```python
from build123d import *

# Parameters (mm, degrees)
SKETCH1_R           = 2.75
BOSS_EXTRUDE1_DEPTH = 6.35
FILLET1_R           = 6.35
CHAMFER1_SIZE       = 3.175


with BuildPart() as part:
    # Sketch1 → Boss-Extrude1 (new body)
    with BuildSketch(Plane.XY):
        with BuildLine():
            ThreePointArc((-19.05, 19.05), (-31.75, 6.35), (-19.05, -6.35))
            Line((-19.05, -6.35), (-19.05, -260.35))
            ThreePointArc((-19.05, -260.35), (-31.75, -273.05), (-19.05, -285.75))
            Line((-19.05, -285.75), (241.3, -285.75))
            ThreePointArc((241.3, -285.75), (254, -273.05), (241.3, -260.35))
            Line((241.3, -260.35), (241.3, -6.35))
            ThreePointArc((241.3, -6.35), (254, 6.35), (241.3, 19.05))
            Line((241.3, 19.05), (-19.05, 19.05))
        make_face()
        with Locations((241.3, 6.35)):
            Circle(SKETCH1_R, mode=Mode.SUBTRACT)
        with Locations((-19.05, -273.05)):
            Circle(SKETCH1_R, mode=Mode.SUBTRACT)
        with Locations((-9.525, -276.225)):
            Circle(SKETCH1_R, mode=Mode.SUBTRACT)
        with Locations((231.775, -276.225)):
            Circle(SKETCH1_R, mode=Mode.SUBTRACT)
        with Locations((241.3, -273.05)):
            Circle(SKETCH1_R, mode=Mode.SUBTRACT)
        with BuildLine():
            Line((-6.35, -247.65), (-6.35, -19.05))
            ThreePointArc((-6.35, -19.05), (6.35, -6.35), (-6.35, 6.35))
            Line((-6.35, 6.35), (228.6, 6.35))
            Line((228.6, 6.35), (228.6, -273.05))
            Line((228.6, -273.05), (-6.35, -273.05))
            ThreePointArc((-6.35, -273.05), (6.35, -260.35), (-6.35, -247.65))
        make_face(mode=Mode.SUBTRACT)
        with Locations((-6.35, -6.35)):
            Circle(SKETCH1_R, mode=Mode.SUBTRACT)
        with Locations((-6.35, -260.35)):
            Circle(SKETCH1_R, mode=Mode.SUBTRACT)
        with Locations((-19.05, 6.35)):
            Circle(SKETCH1_R, mode=Mode.SUBTRACT)
        with Locations((-9.525, 9.525)):
            Circle(SKETCH1_R, mode=Mode.SUBTRACT)
        with Locations((231.775, 9.525)):
            Circle(SKETCH1_R, mode=Mode.SUBTRACT)
    extrude(amount=BOSS_EXTRUDE1_DEPTH)

    # Fillet1
    fillet1_edges = [part.edges().sort_by_distance(p)[0] for p in [
        (228.6, -273.05, 3.175),
        (228.6, 6.35, 3.175),
        (-6.35, 6.35, 3.175),
    ]]
    fillet(fillet1_edges, radius=FILLET1_R)
    fillet1_2_edges = [part.edges().sort_by_distance(p)[0] for p in [
        (-6.35, -273.05, 3.175),
    ]]
    fillet(fillet1_2_edges, radius=FILLET1_R)

    # Chamfer1
    chamfer1_edges = [part.edges().sort_by_distance(p)[0] for p in [
        (-21.8, 6.35, 0),
        (-21.8, -273.05, 0),
        (238.55, 6.35, 0),
        (238.55, -273.05, 0),
        (-9.1, -260.35, 0),
        (-9.1, -6.35, 0),
    ]]
    chamfer(chamfer1_edges, length=CHAMFER1_SIZE)


solid = part.part
```
Input: part model. Units: mm. Frame: model coordinates. A direction names the side the tool comes from. Coordinates: 2 decimals unless noted, no trailing zeros. Write each loop counter-clockwise with the first axis right and the second up, starting at its lowest first coordinate (ties: lowest second). Pieces come first, ordered by that corner, then holes. Notation, with made-up numbers: (-8.75, 49.25) -> (1.25, 49.25) arc R23 ccw to (1.25, 66.25) -> close; hole circle Ø9 at (82.5, 13.5). An arc over 180 degrees is marked (long way). Write each question's results on one line, items separated by ' | '.
Item 1: Section query B-B on y = -73. Return loops of the section in (x, z).
Conclusion:
outline: (-19.05, 0) -> (-6.35, 0) -> (-6.35, 6.35) -> (-19.05, 6.35) -> close; (228.6, 0) -> (241.3, 0) -> (241.3, 6.35) -> (228.6, 6.35) -> close
Item 2: Material intervals for probe 1 along Y at (x, z) = (82.5, 3.25); probe 2 along X at (y, z) = (-220, 4), sorted ascending.
Conclusion:
probe 1: y = -285.75 to -273.05, 6.35 to 19.05 | probe 2: x = -19.05 to -6.35, 228.6 to 241.3
Item 3: Section query A-A on x = 84. Return loops of the section in (y, z), plus the area to 3 significant figures.
Conclusion:
outline: (-285.75, 0) -> (-273.05, 0) -> (-273.05, 6.35) -> (-285.75, 6.35) -> close; (6.35, 0) -> (19.05, 0) -> (19.05, 6.35) -> (6.35, 6.35) -> close | area: 161 mm^2
Item 4: Pin query (flat end, axial travel): pin 1 Ø6.5 at (x, y) = (241.3, -273.05) entering from -Z (3 decimals); pin 2 Ø9 at (x, y) = (241.3, 6.35) entering from -Z (3 decimals); pin 3 Ø1.5 at (y, z) = (-185.5, 5) entering from -X. Return the tip coordinate at first contact, or that it passes through.
Conclusion:
pin 1: stops at z = 2.675 | pin 2: stops at z = 1.425 | pin 3: stops at x = -19.05
Item 5: Section query C-C on z = 5. Count the separate pieces of the cut face and the enclosed holes in it, plus the area to 3 significant figures.
Conclusion:
separate pieces: 1 | enclosed holes: 11 | area: 15,100 mm^2
Item 6: Mould query, pull axis X, two halves, no side actions, for faces 3 (the cylindrical face through (254, -273, 3)), 4 (the flat face through (-19.05, -132, 3)), 5 (the cylindrical face through (6.38, 3.6, 3.22)). Classes: +X half, -X half, draft (parallel to the pull), parting line (faces both ways), or undercut.
Conclusion:
face 3: +X half | face 4: -X half | face 5: undercut
Item 7: Set-up query: faces 1 (the cylindrical face through (6.48, -270.44, 3.22)), 2 (the conical face through (244.1, -272.2, 3)). Return all of +Z, -Z, +X, -X, +Y, -Y with unobstructed straight access to the full face (end or side cutting, diameter ignored); none if empty.
Conclusion:
face 1: +Z, -Z | face 2: -Z
